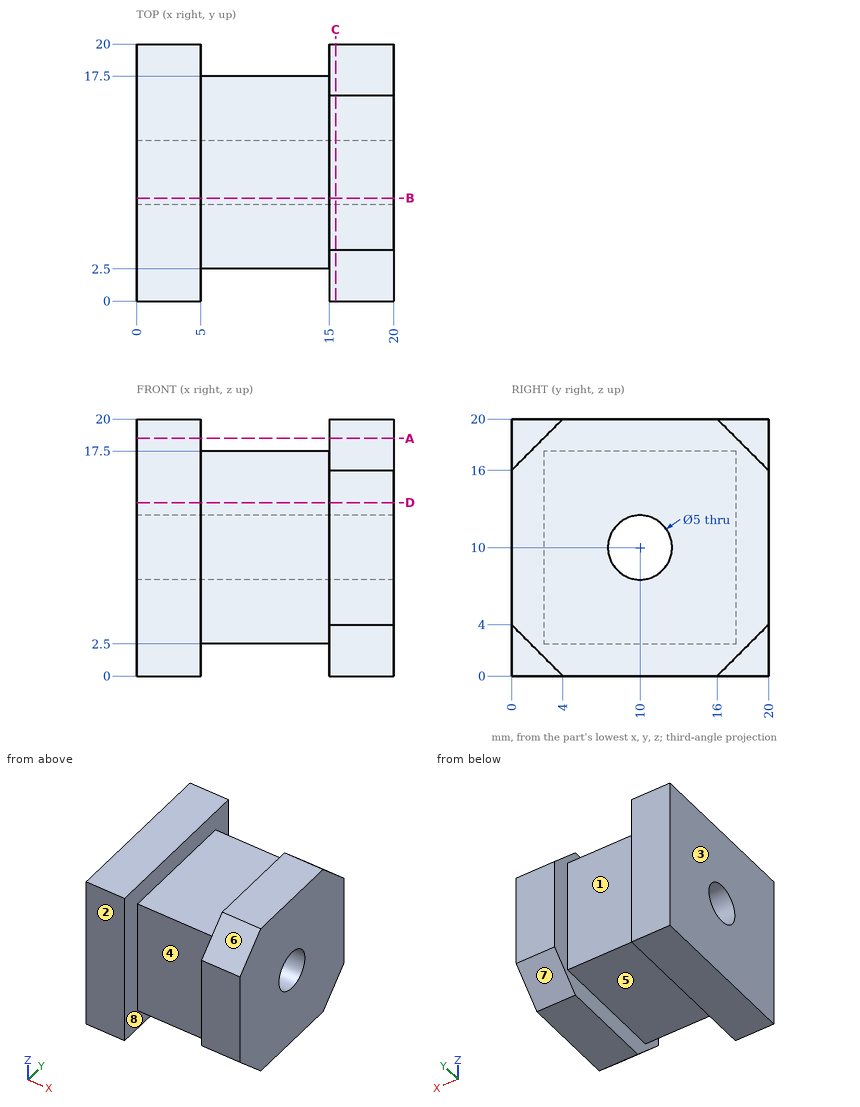
Answer from the drawing. Dimensions are ordinates in mm from the lowest x, y and z of the part. A direction names the side the tool comes from. Give positions to 0.01 mm unless a question says otherwise; leave off trailing zeros. Order: outer loops, then holes, each group sorted by start corner. A loop starts at its lowest first (then second) coordinate and runs counter-clockwise, first axis right, second up.
Item 1: The part is cut by section B-B, the plane y = 8. Give the vertices of the cut face in (x, z).
From the geometry:
outline: (0, 0) - (5, 0) - (5, 2.5) - (15, 2.5) - (15, 0) - (20, 0) - (20, 8.5) - (0, 8.5) - close; (0, 11.5) - (20, 11.5) - (20, 20) - (15, 20) - (15, 17.5) - (5, 17.5) - (5, 20) - (0, 20) - close
Item 2: Find the intervals of material crossed by probe 1 along Z at (x, y) = (4.5, 10); probe 2 along Z at (x, y) = (7.5, 10); probe 3 along X at (y, z) = (2.5, 18), in increasing order.
From the geometry:
probe 1: z = 0 to 7.5, 12.5 to 20
probe 2: z = 2.5 to 7.5, 12.5 to 17.5
probe 3: x = 0 to 5, 15 to 20
Item 3: For a pull along X with two mould halves and no side action, classify the marked faces 1, 2, 3 and 4 as pulls with the +X half, pulls with the -X half, needs draft (parallel to the pull), parting line crosses it, or undercut.
From the geometry:
face 1: undercut
face 2: needs draft
face 3: pulls with the -X half
face 4: undercut
Item 4: The part is cut by section A-A, the plane z = 18.5. Give the vertices of the cut face in (x, y), and give its area (3 significant figures).
From the geometry:
outline: (0, 0) - (5, 0) - (5, 20) - (0, 20) - close; (15, 2.5) - (20, 2.5) - (20, 17.5) - (15, 17.5) - close
area: 175 mm2
Item 5: Which of the six approach directions +Z, -Z, +X, -X, +Y, -Y give full straight-line access (tool end or side, diameter ignored) to the marked faces 5, 6, 7 and 8?
From the geometry:
face 5: -Z, +Y, -Y
face 6: +Z, +X, -Y
face 7: -Z, +X, +Y
face 8: none
Item 6: The part is cut by section C-C, the plane x = 15.5. Give the vertices of the cut face in (y, z).
From the geometry:
outline: (0, 4) - (4, 0) - (16, 0) - (20, 4) - (20, 16) - (16, 20) - (4, 20) - (0, 16) - close; hole circle Ø5 at (10, 10)
Item 7: The part is cut by section D-D, the plane z = 13.5. Give the vertices of the cut face in (x, y), and give its area (3 significant figures).
From the geometry:
outline: (0, 0) - (5, 0) - (5, 2.5) - (15, 2.5) - (15, 0) - (20, 0) - (20, 20) - (15, 20) - (15, 17.5) - (5, 17.5) - (5, 20) - (0, 20) - close
area: 350 mm2
Item 8: Given pin 1 Ø11 at (x, y) = (12.5, 7) entering from +Z; pin 2 Ø5 at (x, z) = (9, 15) entering from +Y; pin 3 Ø2 at (x, z) = (15, 2.5) entering from +Y; pin 4 Ø5 at (x, y) = (10.5, 6.5) entering from -Z, each flat-ended and moving along its own axis, determine where each tip first touches the part or whether it passes through.
From the geometry:
pin 1: stops at z = 20
pin 2: stops at y = 17.5
pin 3: stops at y = 19.5
pin 4: stops at z = 2.5
